```python
from build123d import *

# Parameters (mm, degrees)
F0_W     = 120
F0_H     = 120
F0_R     = 1.5
F1_DEPTH = 2


with BuildPart() as f1:
    # F0 (on Top) → F1 (new body)
    with BuildSketch(Plane.XY):
        with Locations((4.213179, -19.793133)):
            Rectangle(F0_W, F0_H)
        with Locations((-48.08242, -70.88533)):
            Circle(F0_R, mode=Mode.SUBTRACT)
        with Locations((-33.08242, -70.88533)):
            Circle(F0_R, mode=Mode.SUBTRACT)
        with Locations((-48.08242, -55.88533)):
            Circle(F0_R, mode=Mode.SUBTRACT)
        with Locations((-33.08242, -55.88533)):
            Circle(F0_R, mode=Mode.SUBTRACT)
        with Locations((-18.08242, -70.88533)):
            Circle(F0_R, mode=Mode.SUBTRACT)
        with Locations((-3.08242, -70.88533)):
            Circle(F0_R, mode=Mode.SUBTRACT)
        with Locations((-18.08242, -55.88533)):
            Circle(F0_R, mode=Mode.SUBTRACT)
        with Locations((-3.08242, -55.88533)):
            Circle(F0_R, mode=Mode.SUBTRACT)
        with Locations((-48.08242, -40.88533)):
            Circle(F0_R, mode=Mode.SUBTRACT)
        with Locations((-33.08242, -40.88533)):
            Circle(F0_R, mode=Mode.SUBTRACT)
        with Locations((-48.08242, -25.88533)):
            Circle(F0_R, mode=Mode.SUBTRACT)
        with Locations((-33.08242, -25.88533)):
            Circle(F0_R, mode=Mode.SUBTRACT)
        with Locations((-18.08242, -40.88533)):
            Circle(F0_R, mode=Mode.SUBTRACT)
        with Locations((-3.08242, -40.88533)):
            Circle(F0_R, mode=Mode.SUBTRACT)
        with Locations((-18.08242, -25.88533)):
            Circle(F0_R, mode=Mode.SUBTRACT)
        with Locations((-3.08242, -25.88533)):
            Circle(F0_R, mode=Mode.SUBTRACT)
        with Locations((11.91758, -70.88533)):
            Circle(F0_R, mode=Mode.SUBTRACT)
        with Locations((26.91758, -70.88533)):
            Circle(F0_R, mode=Mode.SUBTRACT)
        with Locations((11.91758, -55.88533)):
            Circle(F0_R, mode=Mode.SUBTRACT)
        with Locations((26.91758, -55.88533)):
            Circle(F0_R, mode=Mode.SUBTRACT)
        with Locations((41.91758, -70.88533)):
            Circle(F0_R, mode=Mode.SUBTRACT)
        with Locations((56.91758, -70.88533)):
            Circle(F0_R, mode=Mode.SUBTRACT)
        with Locations((41.91758, -55.88533)):
            Circle(F0_R, mode=Mode.SUBTRACT)
        with Locations((56.91758, -55.88533)):
            Circle(F0_R, mode=Mode.SUBTRACT)
        with Locations((11.91758, -40.88533)):
            Circle(F0_R, mode=Mode.SUBTRACT)
        with Locations((26.91758, -40.88533)):
            Circle(F0_R, mode=Mode.SUBTRACT)
        with Locations((11.91758, -25.88533)):
            Circle(F0_R, mode=Mode.SUBTRACT)
        with Locations((26.91758, -25.88533)):
            Circle(F0_R, mode=Mode.SUBTRACT)
        with Locations((41.91758, -40.88533)):
            Circle(F0_R, mode=Mode.SUBTRACT)
        with Locations((56.91758, -40.88533)):
            Circle(F0_R, mode=Mode.SUBTRACT)
        with Locations((41.91758, -25.88533)):
            Circle(F0_R, mode=Mode.SUBTRACT)
        with Locations((56.91758, -25.88533)):
            Circle(F0_R, mode=Mode.SUBTRACT)
        with Locations((-48.08242, -10.88533)):
            Circle(F0_R, mode=Mode.SUBTRACT)
        with Locations((-33.08242, -10.88533)):
            Circle(F0_R, mode=Mode.SUBTRACT)
        with Locations((-48.08242, 4.11467)):
            Circle(F0_R, mode=Mode.SUBTRACT)
        with Locations((-33.08242, 4.11467)):
            Circle(F0_R, mode=Mode.SUBTRACT)
        with Locations((-18.08242, -10.88533)):
            Circle(F0_R, mode=Mode.SUBTRACT)
        with Locations((-3.08242, -10.88533)):
            Circle(F0_R, mode=Mode.SUBTRACT)
        with Locations((-18.08242, 4.11467)):
            Circle(F0_R, mode=Mode.SUBTRACT)
        with Locations((-3.08242, 4.11467)):
            Circle(F0_R, mode=Mode.SUBTRACT)
        with Locations((-48.08242, 19.11467)):
            Circle(F0_R, mode=Mode.SUBTRACT)
        with Locations((-33.08242, 19.11467)):
            Circle(F0_R, mode=Mode.SUBTRACT)
        with Locations((-48.08242, 34.11467)):
            Circle(F0_R, mode=Mode.SUBTRACT)
        with Locations((-33.08242, 34.11467)):
            Circle(F0_R, mode=Mode.SUBTRACT)
        with Locations((-18.08242, 19.11467)):
            Circle(F0_R, mode=Mode.SUBTRACT)
        with Locations((-3.08242, 19.11467)):
            Circle(F0_R, mode=Mode.SUBTRACT)
        with Locations((-18.08242, 34.11467)):
            Circle(F0_R, mode=Mode.SUBTRACT)
        with Locations((-3.08242, 34.11467)):
            Circle(F0_R, mode=Mode.SUBTRACT)
        with Locations((11.91758, -10.88533)):
            Circle(F0_R, mode=Mode.SUBTRACT)
        with Locations((26.91758, -10.88533)):
            Circle(F0_R, mode=Mode.SUBTRACT)
        with Locations((11.91758, 4.11467)):
            Circle(F0_R, mode=Mode.SUBTRACT)
        with Locations((26.91758, 4.11467)):
            Circle(F0_R, mode=Mode.SUBTRACT)
        with Locations((41.91758, -10.88533)):
            Circle(F0_R, mode=Mode.SUBTRACT)
        with Locations((56.91758, -10.88533)):
            Circle(F0_R, mode=Mode.SUBTRACT)
        with Locations((41.91758, 4.11467)):
            Circle(F0_R, mode=Mode.SUBTRACT)
        with Locations((56.91758, 4.11467)):
            Circle(F0_R, mode=Mode.SUBTRACT)
        with Locations((11.91758, 19.11467)):
            Circle(F0_R, mode=Mode.SUBTRACT)
        with Locations((26.91758, 19.11467)):
            Circle(F0_R, mode=Mode.SUBTRACT)
        with Locations((11.91758, 34.11467)):
            Circle(F0_R, mode=Mode.SUBTRACT)
        with Locations((26.91758, 34.11467)):
            Circle(F0_R, mode=Mode.SUBTRACT)
        with Locations((41.91758, 19.11467)):
            Circle(F0_R, mode=Mode.SUBTRACT)
        with Locations((56.91758, 19.11467)):
            Circle(F0_R, mode=Mode.SUBTRACT)
        with Locations((41.91758, 34.11467)):
            Circle(F0_R, mode=Mode.SUBTRACT)
        with Locations((56.91758, 34.11467)):
            Circle(F0_R, mode=Mode.SUBTRACT)
    extrude(amount=F1_DEPTH)


solid = f1.part
```
The model under review builds one solid part; all positions refer to its coordinate system, in mm. Round coordinates to 2 decimals unless told otherwise and drop trailing zeros.
Item 1: Mouldability with a two-part tool opening along X and no side actions: class faces 1 (the face through (-48.3, -39.4, 1)), 2 (the face through (-49.27, 18.2, 0.99)) as released by +X, released by -X, zero draft, split by the parting line, or undercut.
Determined:
face 1: undercut
face 2: undercut
Item 2: Clearance check with a flat-ended pin moving along its axis: pin 1 Ø2.5 at (x, y) = (56.92, -40.89) entering from +Z. State where the tip first meets the part, or that it passes through.
Determined:
pin 1: passes through
Item 3: Take a section at A-A (z = 0.7). Give the number of separate pieces and of enclosed holes in the cut face, then the cut area to 3 significant figures.
Determined:
separate pieces: 1
enclosed holes: 64
area: 13,900 mm2
